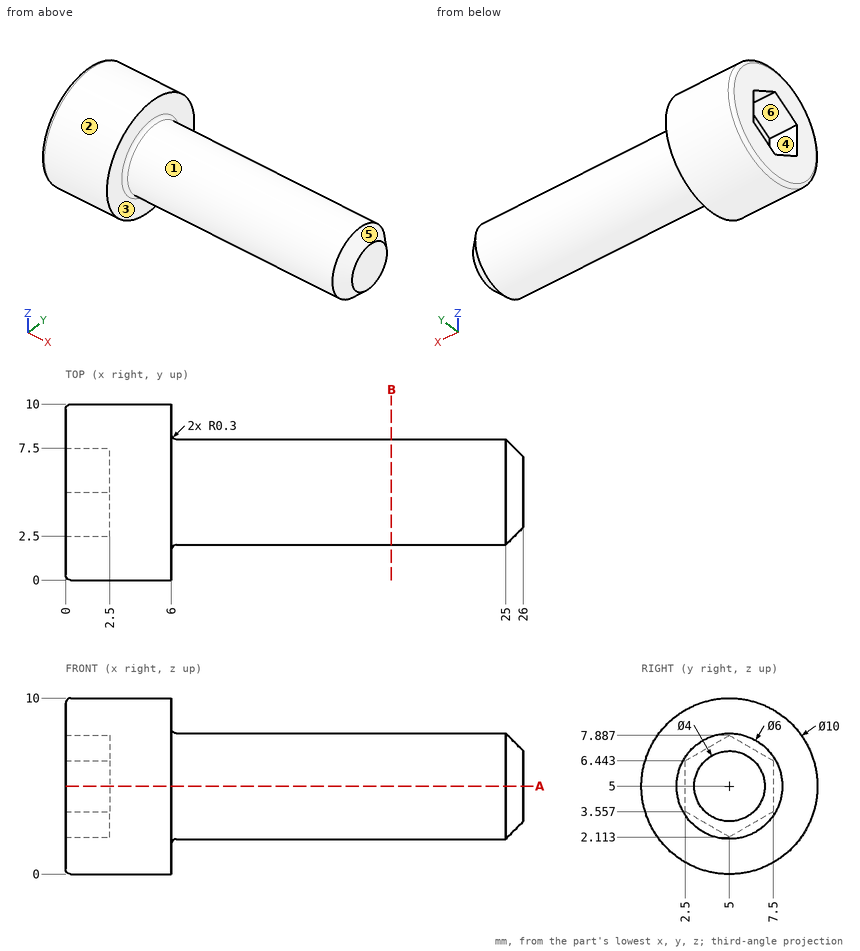
Input: dimensioned drawing with shaded views. Units: mm. Origin: part minimum x, y, z. A direction names the side the tool comes from. Give positions to 0.01 mm unless a question says otherwise; leave off trailing zeros. Order: outer loops, then holes, each group sorted by start corner. A loop starts at its lowest first (then second) coordinate and runs counter-clockwise, first axis right, second up. Notation, with made-up numbers: (-32.5, 50.25) -> (3.5, 50.25) arc R21 cw to (3.5, 85.25) -> close; hole circle Ø11 at (81, 57.25). An arc over 180 degrees is marked (long way). Write item = value, one per line.
Item 1: Contact query for flat-ended pins moving along their axis: pin 1 (1.5 mm diameter, centred on y = 5.5, z = 5.5, fed in from -X); pin 2 (2 mm diameter, centred on x = 12, z = 2, fed in from -Y) (1 decimal); pin 3 (2 mm diameter, centred on x = 16.5, z = 6, fed in from +Y). Output: stop coordinate, or through.
Check result:
pin_1 = 2.5
pin_2 = 2.8
pin_3 = 8
Item 2: Section query B-B (x = 18.5). Output: boundary loops of the cut face in (y, z).
Check result:
outline = circle Ø6 at (5, 5)
Item 3: Ray query, probe 1 along X at (y, z) = (3.75, 5); probe 2 along X at (y, z) = (6, 1); probe 3 along Y at (x, z) = (1.75, 0.5). Return the intervals inside material, ascending.
Check result:
probe_1 = 2.5 to 26
probe_2 = 0 to 6
probe_3 = 2.82 to 7.18
Item 4: Mould query, pull axis Z, two halves, no side actions, for the marked faces 3, 4, 5 and 6. Classes: +Z half, -Z half, draft (parallel to the pull), parting line (faces both ways), or undercut.
Check result:
face_3 = draft
face_4 = undercut
face_5 = parting line
face_6 = undercut
Item 5: Section query A-A (z = 5). Output: boundary loops of the cut face in (x, y).
Check result:
outline = (0, 0.3) arc R0.3 ccw to (0.3, 0) -> (6, 0) -> (6, 1.7) arc R0.3 cw to (6.3, 2) -> (25, 2) -> (26, 3) -> (26, 7) -> (25, 8) -> (6.3, 8) arc R0.3 cw to (6, 8.3) -> (6, 10) -> (0.3, 10) arc R0.3 ccw to (0, 9.7) -> (0, 7.5) -> (2.5, 7.5) -> (2.5, 2.5) -> (0, 2.5) -> close
Item 6: Set-up query: the marked faces 1 and 2. Return all of +Z, -Z, +X, -X, +Y, -Y with unobstructed straight access to the full face (end or side cutting, diameter ignored); none if empty.
Check result:
face_1 = +X
face_2 = +X, -X
